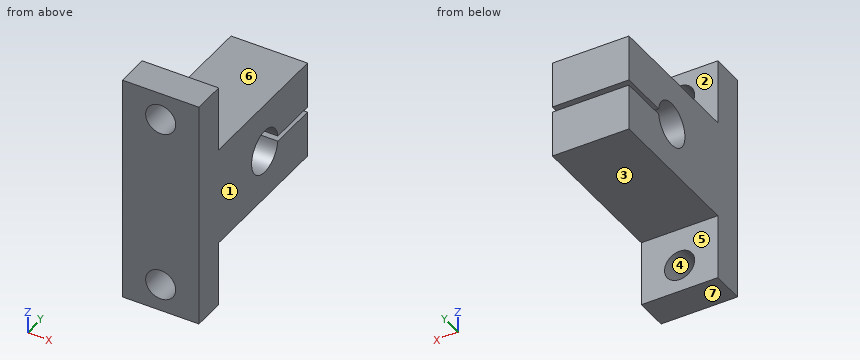
from build123d import *

# Parameters (mm, degrees)
BOSS_EXTRUDE1_DEPTH     = 14
CUT_EXTRUDE1_DEPTH      = 37.959437225
CUT_EXTRUDE1_DEPTH_BACK = 37.959437225
SKETCH2_R               = 2.75


with BuildPart() as part:
    # Sketch1 → Boss-Extrude1 (new body)
    with BuildSketch(Plane(origin=(0, 0, 0), x_dir=(0, 0, -1), z_dir=(1, 0, 0))):
        with BuildLine():
            Line((21, -20), (-21, -20))
            Line((-21, -20), (-21, -14))
            Line((-21, -14), (-9, -14))
            Line((-9, -14), (-9, 13))
            Line((-9, 13), (-0.5, 13))
            Line((-0.5, 13), (-0.5, 3.968626967))
            ThreePointArc((-0.5, 3.968626967), (0, -4), (0.5, 3.968626967))
            Line((0.5, 3.968626967), (0.5, 13))
            Line((0.5, 13), (9, 13))
            Line((9, 13), (9, -14))
            Line((9, -14), (21, -14))
            Line((21, -14), (21, -20))
        make_face()
    extrude(amount=BOSS_EXTRUDE1_DEPTH)

    # Sketch2 → Cut-Extrude1 (cut, two sides: drawn at the far end of the back side and taken through both)
    with BuildSketch(Plane(origin=(0, -14, 0), x_dir=(1, 0, 0), z_dir=(0, 1, 0)).offset(-CUT_EXTRUDE1_DEPTH_BACK)):
        with Locations(Location((7, 16, 0), (0, 0, 270))):
            Circle(SKETCH2_R)
        with Locations(Location((7, -16, 0), (0, 0, 90))):
            Circle(SKETCH2_R)
    extrude(amount=CUT_EXTRUDE1_DEPTH + CUT_EXTRUDE1_DEPTH_BACK, mode=Mode.SUBTRACT)


solid = part.part
The listing builds one solid part. Answer for the finished solid, in the listing's coordinates (mm). Face numbers are marked on the shaded views. A direction names the side the tool comes from. Give positions to 0.01 mm unless a question says otherwise; leave off trailing zeros. Write each loop counter-clockwise with the first axis right and the second up, starting at its lowest first coordinate (ties: lowest second). Pieces come first, ordered by that corner, then holes. Notation, with made-up numbers: (74.25, 22) - (87.25, 22) arc R33 ccw to (87.25, 50) - close; hole circle Ø9 at (52, 58). An arc over 180 degrees is marked (long way). One line per question, with ' | ' between items. Start each with the question number.
1. Determine the mould class of the marked faces 4, 5, 6 and 7 for opening direction Z: +Z half, -Z half, draft (parallel to the pull), parting line (faces both ways), or undercut.
2. Section D-D, the plane x = 12.5 is taken. Determine the outline of the cut face in (y, z).
3. Section B-B, the plane y = 0 is taken. Determine the outline of the cut face in (x, z), then the cut area to 3 significant figures.
4. Section C-C, the plane x = 7 is taken. Determine the outline of the cut face in (y, z).
5. Section A-A, the plane z = -16 is taken. Determine the outline of the cut face in (x, y), then the cut area to 3 significant figures.
6. Given P1, Ø7, axis at x = 7, z = -16, coming from the +Y side; P2, Ø7, axis at x = 5.5, y = 7.5, coming from the +Z side, each flat-ended and moving along its own axis, determine where each tip first touches the part or whether it passes through.
7. For the marked faces 1, 2 and 3, determine the directions among +Z, -Z, +X, -X, +Y, -Y from which every point of the face is accessible in a straight line to the end or side of a thin tool.
8. Straight lines are drawn through the part: line 1 (Z direction, x = 6, y = 7.5); line 2 (Z direction, x = 11, y = 0); line 3 (X direction, y = -15.4, z = -16). For each, find the intervals that lie inside material, in ascending order.
Result:
1) face 4: undercut | face 5: draft | face 6: +Z half | face 7: -Z half
2) outline: (-20, -21) - (-14, -21) - (-14, -9) - (13, -9) - (13, -0.5) - (3.97, -0.5) arc R4 cw (long way) to (3.97, 0.5) - (13, 0.5) - (13, 9) - (-14, 9) - (-14, 21) - (-20, 21) - close
3) outline: (0, -9) - (14, -9) - (14, -4) - (0, -4) - close; (0, 4) - (14, 4) - (14, 9) - (0, 9) - close | area: 140 mm2
4) outline: (-20, -21) - (-14, -21) - (-14, -18.75) - (-20, -18.75) - close; (-20, -13.25) - (-14, -13.25) - (-14, -9) - (13, -9) - (13, -0.5) - (3.97, -0.5) arc R4 cw (long way) to (3.97, 0.5) - (13, 0.5) - (13, 9) - (-14, 9) - (-14, 13.25) - (-20, 13.25) - close; (-20, 18.75) - (-14, 18.75) - (-14, 21) - (-20, 21) - close
5) outline: (0, -20) - (4.25, -20) - (4.25, -14) - (0, -14) - close; (9.75, -20) - (14, -20) - (14, -14) - (9.75, -14) - close | area: 51.0 mm2
6) P1: stops at y = -14 | P2: stops at z = 9
7) face 1: +Z, -Z, +X, +Y, -Y | face 2: +Z, +X, -X, +Y | face 3: -Z, +X, -X, +Y
8) line 1: z = -9 to -0.5, 0.5 to 9 | line 2: z = -9 to -4, 4 to 9 | line 3: x = 0 to 4.25, 9.75 to 14
